from build123d import *

# Parameters (mm, degrees)
PAD_DEPTH       = 1
SKETCH_R        = 7.75
POCKET_DEPTH    = 1.001
POCKET001_DEPTH = 1.001


with BuildPart() as part:
    # Sketch007 → Pad (new body)
    with BuildSketch(Plane.XY):
        with BuildLine():
            Line((13.5, 15.5), (-13.5, 15.5))
            ThreePointArc((-15.469616, 17.152704), (-14.785575, 15.967911), (-13.5, 15.5))
            Line((-15.469616, 17.152704), (-16.153704, 21.03236))
            ThreePointArc((-16.153704, 21.03236), (-17.281843, 22.891476), (-19.369594, 23.5))
            Line((-19.369594, 23.5), (-26.098892, 22.911263))
            ThreePointArc((-26.098892, 22.911263), (-32.808142, 21.113525), (-38.497913, 17.129504))
            Line((-40.313708, 15.313708), (-38.497913, 17.129504))
            ThreePointArc((-40.313708, 15.313708), (-43.782073, 10.122935), (-45, 4))
            Line((-45, 4), (-45, 0))
            Line((-45, 0), (27.5, 0))
            Line((27.5, 0), (27.5, 10.677124))
            ThreePointArc((27.75, 11.338562), (27.564586, 11.030678), (27.5, 10.677124))
            ThreePointArc((27.75, 11.338562), (27.935414, 11.646447), (28, 12))
            Line((28, 18.015221), (28, 12))
            ThreePointArc((28, 18.015221), (26.702361, 20.964331), (23.651377, 22))
            Line((18.502743, 21.549553), (23.651377, 22))
            ThreePointArc((18.502743, 21.549553), (16.73744, 20.772801), (15.809787, 19.081913))
            Line((15.809787, 19.081913), (15.469616, 17.152704))
            ThreePointArc((13.5, 15.5), (14.785575, 15.967911), (15.469616, 17.152704))
        make_face()
        with BuildLine():
            Line((-20, 13), (-17, 13))
            ThreePointArc((-17, 13), (-16.25, 13.75), (-17, 14.5))
            Line((-20, 14.5), (-17, 14.5))
            ThreePointArc((-20, 14.5), (-20.75, 13.75), (-20, 13))
        make_face(mode=Mode.SUBTRACT)
        with BuildLine():
            Line((-1.5, 13), (1.5, 13))
            ThreePointArc((1.5, 13), (2.25, 13.75), (1.5, 14.5))
            Line((-1.5, 14.5), (1.5, 14.5))
            ThreePointArc((-1.5, 14.5), (-2.25, 13.75), (-1.5, 13))
        make_face(mode=Mode.SUBTRACT)
        with BuildLine():
            Line((17, 13), (20, 13))
            ThreePointArc((20, 13), (20.75, 13.75), (20, 14.5))
            Line((17, 14.5), (20, 14.5))
            ThreePointArc((17, 14.5), (16.25, 13.75), (17, 13))
        make_face(mode=Mode.SUBTRACT)
    pad = extrude(amount=PAD_DEPTH)

    # Mirrored: Pad across Sketch007 H_Axis
    add(pad.mirror(Plane.ZX))

    # Sketch (on Face5 of Mirrored) → Pocket (cut, through all)
    with BuildSketch(Plane.XY.offset(1)):
        Circle(SKETCH_R)
    extrude(amount=-POCKET_DEPTH, mode=Mode.SUBTRACT)

    # Sketch008 → Pocket001 (cut, through all)
    with BuildSketch(Plane.XY):
        with BuildLine():
            Line((-41.5, 2.732233), (-41.5, -2.732233))
            ThreePointArc((-41.5, -2.732233), (-39.956709, -5.041932), (-37.232233, -4.5))
            Line((-35.792893, -3.06066), (-37.232233, -4.5))
            ThreePointArc((-35.792893, -3.06066), (-35.57612, -2.736237), (-35.5, -2.353553))
            Line((-35.5, 2.353553), (-35.5, -2.353553))
            ThreePointArc((-35.5, 2.353553), (-35.57612, 2.736237), (-35.792893, 3.06066))
            Line((-37.232233, 4.5), (-35.792893, 3.06066))
            ThreePointArc((-37.232233, 4.5), (-39.956709, 5.041932), (-41.5, 2.732233))
        make_face()
    extrude(amount=POCKET001_DEPTH, mode=Mode.SUBTRACT)


solid = part.part
Can you work these out from the model? Positions are in its coordinate system, mm. A direction names the side the tool comes from. Coordinates: 2 decimals unless noted, no trailing zeros. Write each loop counter-clockwise with the first axis right and the second up, starting at its lowest first coordinate (ties: lowest second). Pieces come first, ordered by that corner, then holes.
Q1. Imagine slicing it at A-A, the plane y = 0. List the corners of the cut face in (x, z) for me, plus the area to 3 significant figures.
Results found:
outline: (-45, 0) - (-41.5, 0) - (-41.5, 1) - (-45, 1) - close; (-35.5, 0) - (-7.75, 0) - (-7.75, 1) - (-35.5, 1) - close; (7.75, 0) - (27.5, 0) - (27.5, 1) - (7.75, 1) - close
area: 51.0 mm2
Q2. For P1, Ø0.5, axis at y = -0.5, z = 0.5, coming from the +X side; P2, Ø0.5, axis at x = 0.5, z = 0.5, coming from the +Y side; P3, Ø3, axis at x = -36, y = 16, coming from the -Z side; P4, Ø0.5, axis at x = 0, z = 0.5, coming from the -Y side, each with a flat end and sliding along its axis, tell me the tip position at first contact or that it passes through.
Results found:
P1: stops at x = 27.5
P2: stops at y = 15.5
P3: stops at z = 0
P4: stops at y = -15.5
Q3. Which directions (+Z, -Z, +X, -X, +Y, -Y) give clear straight access to the entire face, cutting with the end or side of a thin tool? Please do faces 1 (the face through (-9, 0, 0)), 2 (the face through (14.771, -15.955, 0.493)), 3 (the face through (-14.8, 15.98, 0.49)), 4 (the face through (-36.52, 3.79, 0.49)).
Results found:
face 1: -Z, +X, -X, +Y, -Y
face 2: +Z, -Z, -Y
face 3: +Z, -Z, +Y
face 4: +Z, -Z
Q4. Imagine slicing it at B-B, the plane x = 0. List the corners of the cut face in (y, z) for me.
Results found:
outline: (-15.5, 0) - (-14.5, 0) - (-14.5, 1) - (-15.5, 1) - close; (-13, 0) - (-7.75, 0) - (-7.75, 1) - (-13, 1) - close; (7.75, 0) - (13, 0) - (13, 1) - (7.75, 1) - close; (14.5, 0) - (15.5, 0) - (15.5, 1) - (14.5, 1) - close
Q5. Please list where these lines run through material, in increasing order: L1, parallel to Y at x = 0, z = 0.5; L2, parallel to Y at x = 19, z = 0.1; L3, parallel to X at y = 2.5, z = 0.05.
Results found:
L1: y = -15.5 to -14.5, -13 to -7.75, 7.75 to 13, 14.5 to 15.5
L2: y = -21.59 to -14.5, -13 to 13, 14.5 to 21.59
L3: x = -45 to -41.5, -35.51 to -7.34, 7.34 to 27.5
Q6. Imagine slicing it at D-D, the plane z = 0.65. Count the separate pieces of the cut face and the enclosed holes in it, plus the area to 3 significant figures.
Results found:
separate pieces: 1
enclosed holes: 8
area: 2,380 mm2
Q7. Imagine slicing it at C-C, the plane y = -6. List the corners of the cut face in (x, z) for me.
Results found:
outline: (-44.87, 0) - (-4.91, 0) - (-4.91, 1) - (-44.87, 1) - close; (4.91, 0) - (27.5, 0) - (27.5, 1) - (4.91, 1) - close
Q8. If we mould it in two halves opening along Y, with no side actions, what happens to faces 5 (the face through (-39.42, -16.21, 0.49)), 6 (the face through (-39.918, 5.057, 0.493)), 7 (the face through (14.771, 15.955, 0.493))? For each: +Y half, -Y half, draft (parallel to the pull), parting line (faces both ways), or undercut.
Results found:
face 5: -Y half
face 6: undercut
face 7: +Y half
